Here's how the part is built. I have some questions about the finished solid (model axes, mm). A direction names the side the tool comes from. Give positions to 0.01 mm unless a question says otherwise; leave off trailing zeros. Loops run counter-clockwise (first coordinate to the right, second up) from the corner with the lowest first, then second, coordinate; pieces in that order, holes last. Notation, with made-up numbers: (29, -30) - (43, -30) arc R14 cw to (43, -16) - close; hole circle Ø10 at (5.25, -34.75). An arc over 180 degrees is marked (long way). Use one line per item in the form item = value.
from build123d import *

# Parameters (mm, degrees)
SKETCH_R  = 1.65
PAD_DEPTH = 2
FILLET_R  = 6


with BuildPart() as part:
    # Sketch → Pad (new body)
    with BuildSketch(Plane.XY):
        with BuildLine():
            Line((-32, 14), (-32, -14))
            ThreePointArc((-32, -14), (-34.12132, -19.12132), (-29, -17))
            Line((-29, -17), (29, -17))
            ThreePointArc((29, -17), (34.12132, -19.12132), (32, -14))
            Line((32, -14), (32, 14))
            ThreePointArc((32, 14), (34.12132, 19.12132), (29, 17))
            Line((29, 17), (-29, 17))
            ThreePointArc((-29, 17), (-34.12132, 19.12132), (-32, 14))
        make_face()
        with Locations((-32, 17)):
            Circle(SKETCH_R, mode=Mode.SUBTRACT)
        with Locations((-32, -17)):
            Circle(SKETCH_R, mode=Mode.SUBTRACT)
        with Locations((32, -17)):
            Circle(SKETCH_R, mode=Mode.SUBTRACT)
        with Locations((32, 17)):
            Circle(SKETCH_R, mode=Mode.SUBTRACT)
    extrude(amount=PAD_DEPTH)

    # Fillet
    fillet_edges = [part.edges().sort_by_distance(p)[0] for p in [
        (-29, -17, 1),
        (29, -17, 1),
        (32, -14, 1),
        (32, 14, 1),
        (29, 17, 1),
        (-29, 17, 1),
        (-32, 14, 1),
        (-32, -14, 1),
    ]]
    fillet(fillet_edges, radius=FILLET_R)


solid = part.part
(1) For P1, Ø4.5, axis at x = 32, y = -17, coming from the +Z side; P2, Ø2, axis at x = -32, y = -17, coming from the +Z side; P3, Ø1, axis at x = 1.5, z = 1, coming from the +Y side; P4, Ø1, axis at x = 4, z = 1, coming from the -Y side, each with a flat end and sliding along its axis, tell me the tip position at first contact or that it passes through.
Geometry says:
P1 = 2
P2 = through
P3 = 17
P4 = -17
(2) If we section it at C-C (y = 4): List the corners of the cut face in (x, z) for me.
Geometry says:
outline = (-32, 0) - (32, 0) - (32, 2) - (-32, 2) - close
(3) Thinking about a two-plate mould opening in Y: for faces 1 (the cylindrical face through (-27.773, 17.537, 1.014)), 2 (the cylindrical face through (-34.07, 19.17, 0.99)), 3 (the flat face through (0, -17, 1)), which applies, pulls with the +Y half, pulls with the -Y half, needs draft (parallel to the pull), parting line crosses it, or undercut?
Geometry says:
face_1 = pulls with the +Y half
face_2 = undercut
face_3 = pulls with the -Y half
(4) For faces 4 (the cylindrical face through (30.35, 17.07, 0.99)), 5 (the cylindrical face through (-27.773, -17.537, 1.014)), 6 (the cylindrical face through (32.537, 12.773, 1.014)), 7 (the flat face through (-32, 0, 1)), 8 (the cylindrical face through (27.71, 17.51, 1.01)), which set-ups out of +Z, -Z, +X, -X, +Y, -Y let a thin tool reach every point of the face, with its end or its side?
Geometry says:
face_4 = +Z, -Z
face_5 = +Z, -Z, -Y
face_6 = +Z, -Z, +X
face_7 = +Z, -Z, -X
face_8 = +Z, -Z, +Y
(5) If we section it at A-A (z = 0.65): List the corners of the cut face in (x, y) for me, plus the area to 3 significant figures.
Geometry says:
outline = (-34, -14.76) arc R3 ccw (long way) to (-29.76, -19) arc R6 cw to (-25.29, -17) - (25.29, -17) arc R6 cw to (29.76, -19) arc R3 ccw (long way) to (34, -14.76) arc R6 cw to (32, -10.29) - (32, 10.29) arc R6 cw to (34, 14.76) arc R3 ccw (long way) to (29.76, 19) arc R6 cw to (25.29, 17) - (-25.29, 17) arc R6 cw to (-29.76, 19) arc R3 ccw (long way) to (-34, 14.76) arc R6 cw to (-32, 10.29) - (-32, -10.29) arc R6 cw to start; hole circle Ø3.3 at (-32, -17); hole circle Ø3.3 at (-32, 17); hole circle Ø3.3 at (32, -17); hole circle Ø3.3 at (32, 17)
area = 2,240 mm²
(6) If I drill on probe 1 along Y at (x, z) = (8.5, 0.75); probe 2 along X at (y, z) = (4, 0.1); probe 3 along X at (y, z) = (14.5, 1.15), over which ranges is the centre line in solid material (lowest first)?
Geometry says:
probe_1 = -17 to 17
probe_2 = -32 to 32
probe_3 = -33.72 to 33.72
(7) If we section it at B-B (x = -13.5): List the corners of the cut face in (y, z) for me, plus the area to 3 significant figures.
Geometry says:
outline = (-17, 0) - (17, 0) - (17, 2) - (-17, 2) - close
area = 68.0 mm²
